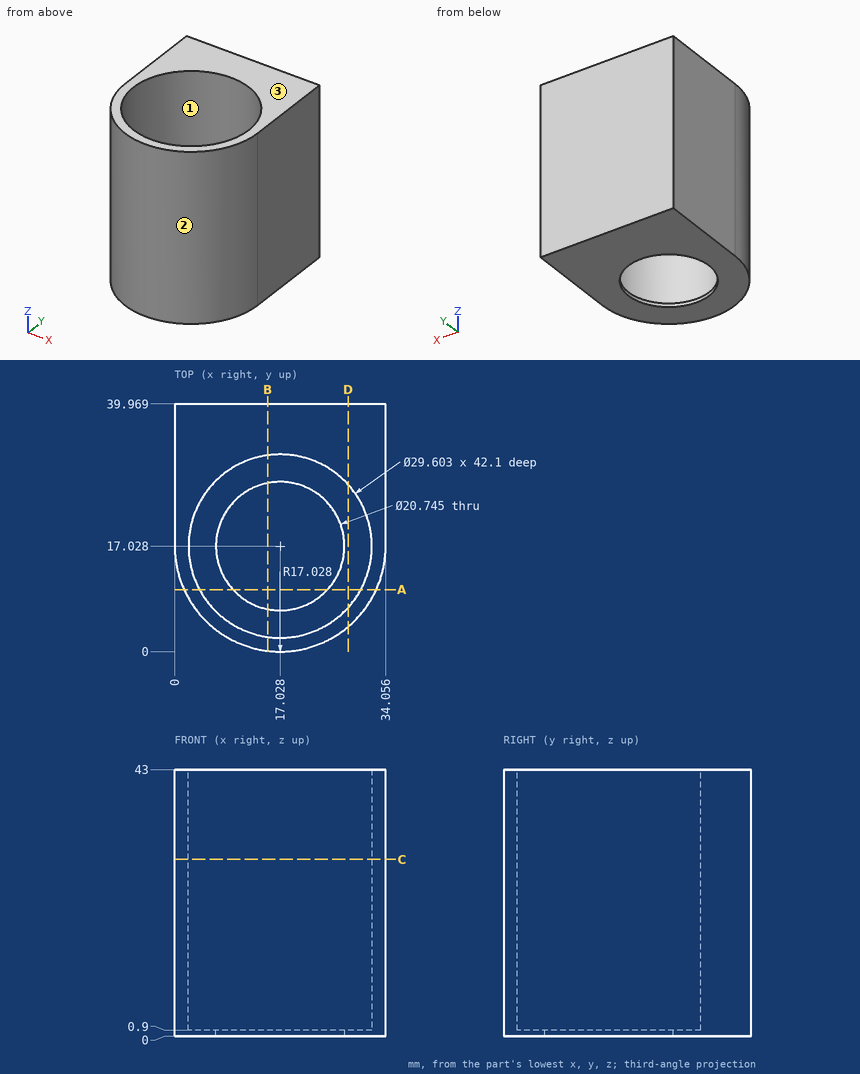
Answer from the drawing. Dimensions are ordinates in mm from the lowest x, y and z of the part. Coordinates: 2 decimals unless noted, no trailing zeros. Loops run counter-clockwise (first coordinate to the right, second up) from the corner with the lowest first, then second, coordinate; pieces in that order, holes last. Notation, with made-up numbers: (1.25, 66.25) -> (25.25, 66.25) arc R20 ccw to (25.25, 95.25) -> close; hole circle Ø4 at (89.25, 82.25). An arc over 180 degrees is marked (long way). Return JSON: item names as keys, results as strings.
Item 1: Find section B-B (x = 15). Determine the outline of the cut face in (y, z) (1 decimal).
Answers:
{"outline": "(0.1, 0) -> (6.9, 0) -> (6.9, 0.9) -> (2.4, 0.9) -> (2.4, 43) -> (0.1, 43) -> close; (27.2, 0) -> (40, 0) -> (40, 43) -> (31.7, 43) -> (31.7, 0.9) -> (27.2, 0.9) -> close"}
Item 2: Find the intervals of material crossed by probe 1 along X at (y, z) = (17, 27); probe 2 along Z at (x, y) = (23, 26); probe 3 along X at (y, z) = (22.5, 7) (1 decimal), in increasing order.
Answers:
{"probe 1": "x = 0 to 2.23, 31.83 to 34.06", "probe 2": "z = 0 to 0.9", "probe 3": "x = 0 to 3.3, 30.8 to 34.1"}
Item 3: Find section A-A (y = 10). Determine the outline of the cut face in (x, z) (1 decimal).
Answers:
{"outline": "(1.5, 0) -> (9.4, 0) -> (9.4, 0.9) -> (4, 0.9) -> (4, 43) -> (1.5, 43) -> close; (24.7, 0) -> (32.5, 0) -> (32.5, 43) -> (30.1, 43) -> (30.1, 0.9) -> (24.7, 0.9) -> close"}
Item 4: Find section D-D (x = 28). Determine the outline of the cut face in (y, z).
Answers:
{"outline": "(4.01, 0) -> (39.97, 0) -> (39.97, 43) -> (26.96, 43) -> (26.96, 0.9) -> (7.09, 0.9) -> (7.09, 43) -> (4.01, 43) -> close"}
Item 5: Find section C-C (z = 28.5). Determine the outline of the cut face in (x, y).
Answers:
{"outline": "(0, 17.03) arc R17.03 ccw to (34.06, 17.03) -> (34.06, 39.97) -> (0, 39.97) -> close; hole circle Ø29.6 at (17.03, 17.03)"}
Item 6: For a pull along X with two mould halves and no side action, classify the marked faces 1, 2 and 3 as +X half, -X half, draft (parallel to the pull), parting line (faces both ways), or undercut.
Answers:
{"face 1": "undercut", "face 2": "parting line", "face 3": "draft"}
Item 7: Flat-ended cylindrical pins translate along their axes: P1, Ø1, axis at y = 23, z = 36, coming from the -X side; P2, Ø2, axis at x = 9.5, y = 24.5, coming from the +Z side; P3, Ø5, axis at y = 5, z = 5, coming from the -X side (1 decimal); P4, Ø6, axis at x = 12, z = 9, coming from the -Y side. Find the tip coordinate at first contact, or state that the pin passes through.
Answers:
{"P1": "stops at x = 0", "P2": "stops at z = 0.9", "P3": "stops at x = 2.9", "P4": "stops at y = 0.12"}
